Autodesk Inventor part; units mm, degrees
ref_plane "Work Plane1" through (29, 0, 0) normal (0, -1, 0) x (1, 0, 0)
ref_plane "YZ Plane" through (0, 0, 0) normal (1, 0, 0) x (0, 1, 0)
ref_plane "XZ Plane" through (0, 0, 0) normal (0, 1, 0) x (-1, 0, 0)
sketch "Szkic1" plane through (0, 0, 0) normal (0, 0, 1) x (1, 0, 0)
  line L0 (-1.1667, 0) -> (20, 0)
  line L1 (20, 0) -> (20, 2.5)
  line L2 (20, 2.5) -> (4, 2.5)
  line L3 (4, 2.5) -> (3.5091, 2.5)
  line L4 (3.5091, 2.5) -> (0, 2.5)
  line L5 (0, 2.5) -> (0, 4.25)
  line L6 (0, 4.25) -> (-5, 4.25)
  line L7 (-5, 4.25) -> (-5, 2.3094)
  line L8 (-5, 2.3094) -> (-2.5, 2.3094)
  line L9 (-2.5, 2.3094) -> (-1.1667, 0)
  line L10 (-10, 0) -> (25, 0)
  line L11 (0, -0.85) -> (0, 5.1)
  line L12 (4, 2.5) -> (0, 2.5) construction
  dimension "d1" = 16
  dimension "d2" = 0.4909
  dimension "d3" = 5
  dimension "d4" = 2.5
  dimension "d5" = 60
  dimension "d6" = 5
  dimension "d7" = 5
  dimension "d8" = 4.6188
  dimension "d9" = 8.5
  dimension "d26" = 20
revolve "Bryła" add sketch "Szkic1" angle 360 about axis through (-1.1667, 0, 0) along (1, 0, 0)
sketch "Szkic2" plane through (-5, 0, 0) normal (-1, 0, 0) x (0, 0, 1)
  circle A0 centre (0, 0) radius 2.3094
  line L0 (0, -5.95) -> (0, 5.95)
  line L1 (-5.95, 0) -> (5.95, 0)
  line L2 (2.3094, 0) -> (1.1547, -2)
  line L3 (1.1547, -2) -> (-1.1547, -2)
  line L4 (-1.1547, -2) -> (-2.3094, 0)
  line L5 (-2.3094, 0) -> (-1.1547, 2)
  line L6 (-1.1547, 2) -> (1.1547, 2)
  line L7 (1.1547, 2) -> (2.3094, 0)
extrude "Szczelina" add sketch "Szkic2" against normal up to next contours L7 A0 | A0 L2 | L6 L0 A0 | A0 L0 L3 | L0 L6 A0 | A0 L3 L0 | L4 A0 | A0 L5
fillet "Zaokrąglenie1" radius 0.5 1 edges at (-5, -4.25, 0)
thread "Gwint"
chamfer "Faza1" distance 0.4908 distance2 0.4908 1 edges at (20, -2.5, 0) measured on face at (20, -0.7379, -0.3873)
ref_plane "Work Plane1" through (29, 0, 0) normal (0, -1, 0) x (1, 0, 0)
fillet "Fillet2" radius 0.1 1 edges at (0, -2.5, 0)
equation "\"d1\" = GEL"
equation "\"d3\" = KOH"
equation "\"d4\" = INTI"
equation "\"d6\" = GD"
equation "\"d7\" = BDM"
equation "\"d8\" = 1.1547 * SW"
equation "\"d9\" = KOD"
equation "\"d26\" = NLG"
equation "\"d30\" = R"
equation "\"d17\" = RR"
equation "\"d13\" = GEL"
equation "\"d15\" = -0.5 * SPD + 0.5 * GD"
equation "\"d16\" = GUL"
equation "\"GD\" = NND"
equation "\"NLG\" = 20"
equation "\"GEL\" = 16"
equation "\"KOD\" = 8.5"
equation "\"KOH\" = NND"
equation "\"INTI\" = 2.5"
equation "\"GAL\" = 0.61345 * PTC"
equation "\"GUL\" = 0.61345 * PTC"
equation "\"BDM\" = NND"
equation "\"SW\" = 4"
equation "\"RR\" = 0.1 * NND"
equation "\"SPD\" = NND - 1.2269 * PTC"
equation "\"R\" = 0.1"
equation "\"PHH\" = 0.13"
equation "\"GD1\" = THREADDIA - 1.2269 * PTC"
equation "\"THREADDIA\" = 5"
equation "\"FAWI\" = 45deg"
equation "\"PTC\" = 0.8"
equation "\"KOH1\" = 4.5"
equation "\"NND\" = 5"
equation "\"TOA\" = 30deg"
equation "\"E0\" = 1.155 * SW"
properties part number "AS 1420 - 1973 - M5 x 20" material "Stal, miękka"
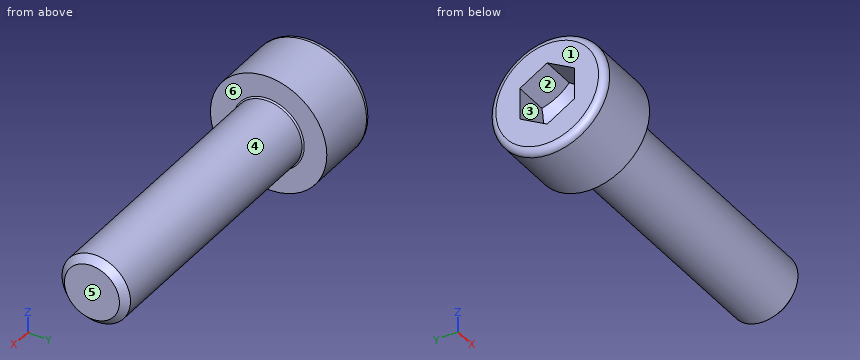
The listing builds one solid part. Answer for the finished solid, in the listing's coordinates (mm). Face numbers are marked on the shaded views. A direction names the side the tool comes from. Coordinates: 2 decimals unless noted, no trailing zeros. Order: outer loops, then holes, each group sorted by start corner. A loop starts at its lowest first (then second) coordinate and runs counter-clockwise, first axis right, second up.
Q1. Consider line 1 (X direction, y = 0, z = 3.75); line 2 (Z direction, x = 12.5, y = -1.5); line 3 (Z direction, x = 12.5, y = 0). Determine where each line is inside the solid, lowest interval first.
Q2. Given P1, Ø1.2, axis at x = -3, z = -0.5, coming from the +Y side; P2, Ø5, axis at x = 14, z = -1, coming from the -Y side; P3, Ø4, axis at x = 16, z = -2.5, coming from the +Y side; P4, Ø1.5, axis at x = 0, y = -1.5, coming from the +Z side, each flat-ended and moving along its own axis, determine where each tip first touches the part or whether it passes through.
Q3. A cutting plane is placed at B-B, the plane x = -2. Write down the section's boundary in (y, z), and give its area (3 significant figures).
Q4. Which of the six approach directions +Z, -Z, +X, -X, +Y, -Y give full straight-line access (tool end or side, diameter ignored) to the marked faces 5 and 6?
Q5. For a pull along Y with two mould halves and no side action, classify the marked faces 1, 2, 3 and 4 as pulls with the +Y half, pulls with the -Y half, needs draft (parallel to the pull), parting line crosses it, or undercut.
Q6. A cutting plane is placed at A-A, the plane x = 13.5. Write down the section's boundary in (y, z), and give its area (3 significant figures).
Answers follow:
1. line 1: x = -5 to 0
1. line 2: z = -2 to 2
1. line 3: z = -2.5 to 2.5
2. P1: stops at y = 4.25
2. P2: stops at y = -2.5
2. P3: stops at y = 2.45
2. P4: stops at z = 4.18
3. outline: circle Ø8.5 at (0, 0); hole circle Ø2.89 at (0, 0)
3. area: 50.2 mm2
4. face 5: +Z, -Z, +X, +Y, -Y
4. face 6: +X
5. face 1: needs draft
5. face 2: undercut
5. face 3: undercut
5. face 4: parting line crosses it
6. outline: circle Ø5 at (0, 0)
6. area: 19.6 mm2
